Check sheet for the modelled part. Datum: model origin and axes. Units: mm. A direction names the side the tool comes from. Give positions to 0.01 mm unless a question says otherwise; leave off trailing zeros. Loops run counter-clockwise (first coordinate to the right, second up) from the corner with the lowest first, then second, coordinate; pieces in that order, holes last. Notation, with made-up numbers: (-26.5, 16) -> (-20.5, 16) arc R19 ccw to (-20.5, 51) -> close; hole circle Ø5 at (14.25, 77.25). An arc over 180 degrees is marked (long way). Write each question's results on one line, items separated by ' | '. Start each with the question number.
Item 1: Gauge pin test, flat ends, axial feed: pin 1 Ø1.5 at (y, z) = (-31.5, 1.5) entering from -X; pin 2 Ø1.5 at (x, z) = (-77, 1.5) entering from +Y; pin 3 Ø0.9 at (x, z) = (-13, 2) entering from -Y. Record the tip position at first contact, or that the pin passes through.
Item 2: Mould release check, pull along X, two halves, no side actions. Record for faces 1 (the face through (-56.169, -19.374, 1.479)), 2 (the face through (-29, -32.393, 2)), 3 (the face through (-12, -31, 1)): pulls with the +X half, pulls with the -X half, needs draft (parallel to the pull), parting line crosses it, or undercut.
Item 3: Access from +Z, -Z, +X, -X, +Y, -Y to the whole of each face (thin tool, end or side, straight path). Record for faces 4 (the face through (-33.1, -31, 1)), 5 (the face through (-34, 8, 3)).
Item 4: Cross-section at A-A on y = 51. Enter the section's corners in (x, z).
Item 5: Cross-section at B-B on x = -55.5. Enter the section's corners in (y, z), then the cut area to 3 significant figures.
Item 6: Scan lines: line 1 along Y through (x, z) = (-75, 1.8); line 2 along Y through (x, z) = (-71.5, 0.4); line 3 along X through (y, z) = (42.5, 1). Record each from-to range of solid material in increasing order.
from build123d import *

# Parameters (mm, degrees)
PAD_DEPTH           = 3
FILLET_R            = 5
FILLET001_R         = 5
SKETCH001_W         = 2.9
SKETCH001_H         = 3
PAD001_DEPTH        = 3
LINEARPATTERN_COUNT = 6
LINEARPATTERN_PITCH = 6


with BuildPart() as part:
    # Sketch → Pad (new body)
    with BuildSketch(Plane.XY):
        with BuildLine():
            Line((-80, -29.392822), (0, -29.392822))
            Line((-3.899435, -25.004208), (0, -29.392822))
            ThreePointArc((-27.274722, 30.700125), (-20.212397, 0.907029), (-3.899435, -25.004208))
            Line((-30, 70.607178), (-27.274722, 30.700125))
            Line((-30, 70.607178), (-40, 70.607178))
            Line((-40, 70.607178), (-46.966643, 0))
            ThreePointArc((-75, -28.392822), (-55.956109, -19.159977), (-46.966643, 0))
            Line((-75, -28.392822), (-80, -28.392822))
            Line((-80, -28.392822), (-80, -29.392822))
        make_face()
    extrude(amount=PAD_DEPTH)

    # Fillet
    fillet_edges = [part.edges().sort_by_distance(p)[0] for p in [
        (-40, 70.607178, 1.5),
    ]]
    fillet(fillet_edges, radius=FILLET_R)

    # Fillet001
    fillet001_edges = [part.edges().sort_by_distance(p)[0] for p in [
        (-30, 70.607178, 1.5),
    ]]
    fillet(fillet001_edges, radius=FILLET001_R)

    # Sketch001 → Pad001 (new body)
    with BuildSketch(Plane.XZ.offset(29.392822)):
        with Locations((-40.55, 1.5)):
            Rectangle(SKETCH001_W, SKETCH001_H)
    pad001 = extrude(amount=PAD001_DEPTH)

    # LinearPattern: Pad001 ×6
    with Locations(*[(i * LINEARPATTERN_PITCH, 0, 0) for i in range(1, LINEARPATTERN_COUNT)]):
        add(pad001)


solid = part.part
Answer sheet:
1) pin 1: stops at x = -42 | pin 2: stops at y = -28.39 | pin 3: stops at y = -29.39
2) face 1: pulls with the -X half | face 2: needs draft | face 3: undercut
3) face 4: +Z, -Z, -Y | face 5: +Z, +X, -X, +Y, -Y
4) outline: (-41.93, 0) -> (-28.66, 0) -> (-28.66, 3) -> (-41.93, 3) -> close
5) outline: (-29.39, 0) -> (-18.69, 0) -> (-18.69, 3) -> (-29.39, 3) -> close | area: 32.1 mm²
6) line 1: y = -29.39 to -28.39 | line 2: y = -29.39 to -27.8 | line 3: x = -42.77 to -28.08
